```python
from build123d import *

# Parameters (mm, degrees)
F1_DEPTH   = 25.4
F4_D       = 5.25
F4_ON_F3_D = 5.25
F5_R       = 5.08


with BuildPart() as f1:
    # F0 (on Front) → F1 (new body)
    with BuildSketch(Plane.XZ):
        with BuildLine():
            Line((0, 63.5), (0, 0))
            Line((0, 0), (76.2, 0))
            Line((76.2, 0), (76.2, 63.5))
            Line((76.2, 63.5), (52.578, 63.5))
            Line((52.578, 63.5), (52.578, 25.654))
            ThreePointArc((52.578, 25.654), (38.1, 11.176), (23.622, 25.654))
            Line((23.622, 25.654), (23.622, 63.5))
            Line((23.622, 63.5), (0, 63.5))
        make_face()
    extrude(amount=F1_DEPTH)

    # F4 (through all)
    with Locations(Plane.XY.offset(63.5)):
        with Locations((11.811, -12.7)):
            Hole(F4_D / 2)

    # F4 on F3 (through all)
    with Locations(Plane.XY.offset(63.5)):
        with Locations((64.389, -12.7)):
            Hole(F4_ON_F3_D / 2)

    # F5
    f5_edges = [f1.edges().sort_by_distance(p)[0] for p in [
        (23.622, -12.7, 63.5),
        (52.578, -12.7, 63.5),
    ]]
    fillet(f5_edges, radius=F5_R)


solid = f1.part
```
Source: CAD feature listing. Evaluate the final solid. Frame: model axes, mm. A direction names the side the tool comes from. Give positions to 0.01 mm unless a question says otherwise; leave off trailing zeros. Write each loop counter-clockwise with the first axis right and the second up, starting at its lowest first coordinate (ties: lowest second). Pieces come first, ordered by that corner, then holes.
1. Section query B-B (y = -12.7). Return the cut outline in (x, z), then the cut area to 3 significant figures.
2. Access query for faces 5 (the face through (21, 0, 32)), 6 (the face through (54.106, -12.878, 62.051)). Directions: +Z, -Z, +X, -X, +Y, -Y. A direction counts if a zero-diameter tool reaches every point of the face in a straight line with its end or side. Return the directions, or none.
3. Pull-direction query (X, two-part tool) for faces 1 (the face through (0, -13, 32)), 2 (the face through (21, -25.4, 32)), 3 (the face through (76.2, -13, 31)), 4 (the face through (61.885, -11.912, 31.305)); classes: +X half, -X half, draft (parallel to the pull), parting line (faces both ways), or undercut.
4. Section query A-A (z = 40). Return the cut outline in (x, y) (3 decimals), then the cut area to 3 significant figures.
5. Section query C-C (x = 10.5). Return the cut outline in (y, z), then the cut area to 3 significant figures.
6. Material intervals for line 1 along X through (y, z) = (-9.75, 41); line 2 along Y through (x, z) = (13, 15); line 3 along X through (y, z) = (-15.75, 17.5), sorted ascending.
7. Section query D-D (z = 22.5). Return the cut outline in (x, y) (3 decimals), then the cut area to 3 significant figures.
Output values:
1. outline: (0, 0) - (9.19, 0) - (9.19, 63.5) - (0, 63.5) - close; (14.44, 0) - (61.76, 0) - (61.76, 63.5) - (57.66, 63.5) arc R5.08 ccw to (52.58, 58.42) - (52.58, 25.65) arc R14.48 cw to (23.62, 25.65) - (23.62, 58.42) arc R5.08 ccw to (18.54, 63.5) - (14.44, 63.5) - close; (67.01, 0) - (76.2, 0) - (76.2, 63.5) - (67.01, 63.5) - close
1. area: 2,740 mm2
2. face 5: +Z, -Z, +X, -X, +Y
2. face 6: +Z, +Y, -Y
3. face 1: -X half
3. face 2: draft
3. face 3: +X half
3. face 4: undercut
4. outline: (0, -25.4) - (23.622, -25.4) - (23.622, 0) - (0, 0) - close; (52.578, -25.4) - (76.2, -25.4) - (76.2, 0) - (52.578, 0) - close; hole circle Ø5.25 at (11.811, -12.7); hole circle Ø5.25 at (64.389, -12.7)
4. area: 1,160 mm2
5. outline: (-25.4, 0) - (-14.97, 0) - (-14.97, 63.5) - (-25.4, 63.5) - close; (-10.43, 0) - (0, 0) - (0, 63.5) - (-10.43, 63.5) - close
5. area: 1,320 mm2
6. line 1: x = 0 to 23.62, 52.58 to 76.2
6. line 2: y = -25.4 to -15.04, -10.36 to 0
6. line 3: x = 0 to 26.14, 50.06 to 76.2
7. outline: (0, -25.4) - (23.97, -25.4) - (23.97, 0) - (0, 0) - close; (52.23, -25.4) - (76.2, -25.4) - (76.2, 0) - (52.23, 0) - close; hole circle Ø5.25 at (11.811, -12.7); hole circle Ø5.25 at (64.389, -12.7)
7. area: 1,170 mm2
